Verification items for the finished model (mm, model axes). A direction names the side the tool comes from. Give positions to 0.01 mm unless a question says otherwise; leave off trailing zeros. Loops run counter-clockwise (first coordinate to the right, second up) from the corner with the lowest first, then second, coordinate; pieces in that order, holes last. Notation, with made-up numbers: (67, 74.5) - (117, 74.5) arc R17 ccw to (117, 94.5) - close; hole circle Ø1 at (37.25, -29). An arc over 180 degrees is marked (long way). Put each result on its own line as item: value. Start each with the question number.
```python
from build123d import *

# Parameters (mm, degrees)
CROQUIS1_W              = 390
CROQUIS1_H              = 50.8
SALIENTE_EXTRUIR1_DEPTH = 3
CROQUIS2_W              = 390
CROQUIS2_H              = 3
SALIENTE_EXTRUIR2_DEPTH = 47.8
CROQUIS3_W              = 3
CROQUIS3_H              = 23.9
CORTAR_EXTRUIR1_DEPTH   = 390
CORTAR_EXTRUIR2_REACH   = 205.296
CROQUIS4_W              = 390
CROQUIS4_H              = 25.4


with BuildPart() as part:
    # Croquis1 → Saliente-Extruir1 (new body)
    with BuildSketch(Plane.XY):
        Rectangle(CROQUIS1_W, CROQUIS1_H)
    extrude(amount=SALIENTE_EXTRUIR1_DEPTH)

    # Croquis2 → Saliente-Extruir2 (add)
    with BuildSketch(Plane.XY.offset(3)):
        Rectangle(CROQUIS2_W, CROQUIS2_H)
    extrude(amount=SALIENTE_EXTRUIR2_DEPTH)

    # Croquis3 → Cortar-Extruir1 (cut)
    with BuildSketch(Plane.ZY.offset(195)):
        with Locations((1.5, 13.45)):
            Rectangle(CROQUIS3_W, CROQUIS3_H)
    extrude(amount=-CORTAR_EXTRUIR1_DEPTH, mode=Mode.SUBTRACT)

    # Croquis4 → Cortar-Extruir2 (cut, up to next)
    with BuildSketch(Plane(origin=(0, 1.5, 0), x_dir=(1, 0, 0), z_dir=(0, 1, 0)), mode=Mode.PRIVATE) as cortar_extruir2_sk1:
        with Locations((0, -38.1)):
            Rectangle(CROQUIS4_W, CROQUIS4_H)
    cortar_extruir2_tool1 = extrude(cortar_extruir2_sk1.sketch, amount=-CORTAR_EXTRUIR2_REACH, mode=Mode.PRIVATE) & part.part
    add(cortar_extruir2_tool1.solids().sort_by_distance((0, 1.5, 38.1))[0], mode=Mode.SUBTRACT)


solid = part.part
```
1) Depth check by flat-ended pin: P1, Ø11, axis at x = -66, z = 11.5, coming from the -Y side; P2, Ø12, axis at y = -2, z = 9, coming from the -X side; P3, Ø2, axis at x = 49.5, y = -16.5, coming from the +Z side. Enter the tip coordinate at first touch or a pass-through.
2) Section check B-B, the plane y = -11. Enter the section's corners in (x, z), plus the area to 3 significant figures.
3) Scan lines: line 1 along Z through (x, y) = (0, -3.5); line 2 along Y through (x, z) = (64.5, 24.25). Record each from-to range of solid material in increasing order. Write a range as from..to.
4) Set-up check for faces 1 (the face through (-195, -7, 2)), 2 (the face through (-3, -1.5, 14)): record each of +Z, -Z, +X, -X, +Y, -Y from which the full face is reachable in a straight line by a thin tool's end or side.
5) Section check C-C, the plane z = 6.75. Enter the section's corners in (x, y).
6) Section check A-A, the plane x = 23. Enter the section's corners in (y, z), plus the area to 3 significant figures.
Results are:
1. P1: stops at y = -1.5
1. P2: stops at x = -195
1. P3: stops at z = 3
2. outline: (-195, 0) - (195, 0) - (195, 3) - (-195, 3) - close
2. area: 1,170 mm2
3. line 1: z = 0..3
3. line 2: y = -1.5..1.5
4. face 1: +Z, -Z, -X, +Y, -Y
4. face 2: +Z, +X, -X, -Y
5. outline: (-195, -1.5) - (195, -1.5) - (195, 1.5) - (-195, 1.5) - close
6. outline: (-25.4, 0) - (1.5, 0) - (1.5, 25.4) - (-1.5, 25.4) - (-1.5, 3) - (-25.4, 3) - close
6. area: 148 mm2
